Autodesk Inventor part; units mm, degrees
ref_plane "YZ Plane" through (0, 0, 0) normal (1, 0, 0) x (0, 1, 0)
ref_plane "XZ Plane" through (0, 0, 0) normal (0, 1, 0) x (-1, 0, 0)
ref_plane "XY Plane" through (0, 0, 0) normal (0, 0, 1) x (1, 0, 0)
sketch "Sketch1" plane through (0, 0, 0) normal (1, 0, 0) x (0, 1, 0)
  line L0 (0, 0) -> (22.86, 0)
  line L1 (22.86, 0) -> (22.86, -22.86)
  line L2 (22.86, -22.86) -> (0, -22.86)
  line L3 (0, -22.86) -> (0, 0)
  line L4 (0, -22.86) -> (15.24, -22.86)
  line L5 (0, -22.86) -> (15.24, -22.86) construction
  line L6 (15.24, -22.86) -> (15.24, -27.94)
  line L7 (15.24, -27.94) -> (17.78, -27.94)
  line L8 (17.78, -27.94) -> (17.78, -22.86)
  line L9 (17.78, 0) -> (17.78, 5.08)
  line L10 (17.78, 5.08) -> (15.24, 5.08)
  line L11 (15.24, 5.08) -> (15.24, 0)
  line L12 (17.9128, 0) -> (15.0818, 0)
  line L13 (15.0818, 5.3336) -> (17.9128, 5.3336)
  line L14 (17.9128, -22.86) -> (15.0818, -22.86)
  line L15 (15.0818, -28.1853) -> (17.9128, -28.1853)
  line L16 (17.9128, 0.0837) -> (17.9128, 5.3336)
  line L17 (15.0818, 0.0837) -> (15.0818, 5.3336)
  line L18 (15.0818, 0.0837) -> (-0.2071, 0.0837)
  line L19 (-0.2071, 0.0837) -> (-0.2071, -23.0588)
  line L20 (-0.2071, -23.0588) -> (15.0818, -23.0588)
  line L21 (15.0818, -23.0588) -> (15.0818, -28.1853)
  line L22 (17.9128, -28.1853) -> (17.9128, -23.0588)
  line L23 (17.9128, -23.0588) -> (22.86, -23.0588)
  line L24 (22.86, -23.0588) -> (22.86, -29.4177)
  line L25 (22.86, -29.4177) -> (-6.35, -29.4177)
  line L26 (22.86, 0.0837) -> (17.9128, 0.0837)
  line L27 (22.86, 0.0837) -> (22.86, 6.4337)
  line L28 (22.86, 6.4337) -> (-6.35, 6.4337)
  line L29 (-6.35, -29.4177) -> (-6.35, 6.4337)
  dimension "d0" = 22.86
  dimension "d1" = 22.86
  dimension "d4" = 5.08
  dimension "d5" = 2.54
  dimension "d6" = 5.08
  dimension "d7" = 2.54
  dimension "d9" = 29.21
  dimension "d11" = 6.35
extrude "Extrusion1" add sketch "Sketch1" along normal blind 12.7 contours L17 L18 L19 L20 L21 L15 L22 L23 L24 L25 L29 L28 L27 L26 L16 L13
sketch "Sketch2" plane through (12.7, 0, 0) normal (1, 0, 0) x (0, 0, -1)
  line L0 (-6.4337, 22.86) -> (-6.4337, -6.35)
  line L1 (29.4177, 22.86) -> (23.0588, 22.86)
  line L2 (-6.4337, -6.35) -> (29.4177, -6.35)
  line L3 (29.4177, -6.35) -> (29.4177, 22.86)
  line L4 (29.4177, 22.86) -> (-6.4337, 22.86)
  line L5 (-6.4337, 22.86) -> (-6.4337, -6.35)
  point P0 (0, 0)
  dimension "d16" = 29.21
  dimension "d17" = 35.8513
extrude "Extrusion2" add sketch "Sketch2" along normal blind 2.54
sketch "Sketch3" plane through (0, 0, 0) normal (-1, 0, 0) x (0, 0, 1)
  line L0 (-29.4177, -6.35) -> (-29.4177, 22.86)
  line L1 (6.4337, -6.35) -> (-29.4177, -6.35)
  line L2 (-29.4177, 0) -> (6.4337, 0)
  line L3 (6.4337, 0) -> (6.4337, -6.35)
  line L4 (6.4337, -6.35) -> (-29.4177, -6.35)
  line L5 (-29.4177, -6.35) -> (-29.4177, 0)
  point P0 (0, 0)
extrude "Extrusion3" add sketch "Sketch3" along normal blind 25.4
sketch "Sketch4" plane through (-25.4, 0, 0) normal (-1, 0, 0) x (0, 0, 1)
  line L0 (6.4337, -6.35) -> (-29.4177, -6.35)
  line L1 (6.4337, 22.86) -> (6.4337, -6.35)
  line L2 (-29.4177, -6.35) -> (6.4337, -6.35)
  line L3 (6.4337, -6.35) -> (6.4337, 22.86)
  line L4 (-29.4177, 22.86) -> (-29.4177, -6.35)
  line L5 (6.4337, 32.258) -> (-29.4177, 32.258)
  line L6 (-29.4177, 32.258) -> (-29.4177, 22.86)
  line L7 (-29.4177, 32.258) -> (-7.1927, 32.258)
  line L8 (-7.1927, 32.258) -> (-11.6377, 32.258)
  line L9 (-29.4177, 22.86) -> (6.4337, 22.86)
  line L10 (-11.6377, 32.258) -> (-9.4152, 32.258)
  line L11 (-9.4152, 22.86) -> (-11.6377, 22.86)
  line L12 (-9.4152, 22.86) -> (-13.8602, 22.86)
  line L13 (-13.8602, 22.86) -> (-13.8602, 32.258)
  line L14 (-13.8602, 32.258) -> (-9.4152, 32.258)
  line L15 (-27.8895, 28.6463) -> (-14.6164, 28.6463)
  line L16 (-14.6164, 28.6463) -> (-14.6164, 25.8191)
  line L17 (-14.6164, 25.8191) -> (-27.8895, 25.8191)
  line L18 (-27.8895, 25.8191) -> (-27.8895, 28.6463)
  line L19 (-8.2851, 28.6463) -> (5.4248, 28.6463)
  line L20 (5.4248, 28.6463) -> (5.4248, 25.8191)
  line L21 (5.4248, 25.8191) -> (-8.2851, 25.8191)
  line L22 (-8.2851, 25.8191) -> (-8.2851, 28.6463)
  line L23 (-8.2851, 28.6463) -> (5.4248, 28.6463)
  line L24 (5.4248, 28.6463) -> (5.4248, 25.8191)
  line L25 (5.4248, 25.8191) -> (-8.2851, 25.8191)
  line L26 (-8.2851, 25.8191) -> (-8.2851, 28.6463)
  line L27 (6.4337, 32.258) -> (-9.4152, 32.258)
  line L28 (-9.4152, 32.258) -> (-9.4152, 22.86)
  line L29 (-9.4152, 22.86) -> (6.4337, 22.86)
  line L30 (6.4337, 22.86) -> (6.4337, 32.258)
  line L31 (-29.4177, -6.35) -> (-29.4177, 22.86)
  line L32 (0.0837, 22.86) -> (6.4337, 22.86)
  line L33 (-29.4177, 22.86) -> (6.4337, 22.86)
  line L34 (6.4337, 22.86) -> (6.4337, 32.258)
  line L35 (6.4337, 32.258) -> (-29.4177, 32.258)
  line L36 (-29.4177, 22.86) -> (-29.4177, 32.258)
  point P0 (0, 0)
  dimension "d21" = 22.225
  dimension "d23" = 2.2225
  dimension "d24" = 4.445
extrude "Extrusion7" add sketch "Sketch4" along normal blind 12.7 contours L0 L4 L9 L1 | L9 L28 L5 L30 | L6 L5 L13 L9
sketch "Sketch6" plane through (-25.4, 32.258, -13.8602) normal (0, 1, 0) x (1, 0, 0)
  line L0 (0, 15.5575) -> (-12.7, 15.5575)
  line L1 (0, -20.2938) -> (-12.7, -20.2938)
  line L2 (-12.7, 15.5575) -> (0, 15.5575)
  line L3 (0, 15.5575) -> (0, -20.2938)
  line L4 (0, -20.2938) -> (-12.7, -20.2938)
  line L5 (-12.7, -20.2938) -> (-12.7, 15.5575)
  point P0 (25.4, -13.8602)
extrude "Extrusion8" add sketch "Sketch6" along normal blind 2.54
sketch "Sketch7" plane through (0, 22.86, 6.4337) normal (0, 0, 1) x (1, 0, 0)
  line L0 (0, 0) -> (15.24, 0)
  line L1 (-38.1, -29.21) -> (-38.1, 11.938)
  line L2 (15.24, 0) -> (-38.1, 0)
  line L3 (-38.1, 0) -> (-38.1, -29.21)
  line L4 (-38.1, -29.21) -> (15.24, -29.21)
  line L5 (15.24, -29.21) -> (15.24, 0)
  point P0 (0, -22.86)
extrude "Extrusion9" add sketch "Sketch7" along normal blind 2.54
sketch "Sketch8" plane through (0, 22.86, -23.0588) normal (0, 1, 0) x (1, 0, 0)
  line L0 (15.24, -32.0324) -> (-38.1, -32.0324)
  line L1 (-12.8761, -32.0324) -> (9.9839, -32.0324)
  line L2 (-12.8761, -47.2724) -> (-12.8761, -32.0324)
  line L3 (9.9839, -47.2724) -> (15.24, -47.2724)
  line L4 (15.24, -32.0324) -> (9.9839, -32.0324)
  line L5 (9.9839, -32.0324) -> (9.9839, -47.2724)
  line L6 (-12.8761, -47.2724) -> (-18.1339, -47.2724)
  line L7 (-18.1339, -32.0324) -> (-12.8761, -32.0324)
  line L8 (-12.8761, -32.0324) -> (-12.8761, -47.2724)
  line L9 (9.9839, -32.0324) -> (15.24, -32.0324)
  line L10 (15.24, -47.2724) -> (9.9839, -47.2724)
  line L11 (9.9839, -47.2724) -> (9.9839, -32.0324)
  line L12 (-18.1339, -32.0324) -> (15.24, -32.0324)
  line L13 (15.24, -32.0324) -> (15.24, -47.2724)
  line L14 (15.24, -32.0324) -> (9.9839, -32.0324)
  line L15 (-18.1339, -47.2724) -> (-18.1339, -32.0324)
  line L16 (-12.8761, -32.0324) -> (-18.1339, -32.0324)
  point P0 (0, -23.0588)
  dimension "d37" = 22.86
  dimension "d39" = 5.2578
extrude "Extrusion11" add sketch "Sketch8" against normal blind 29.21
sketch "Sketch9" plane through (-18.1339, 22.86, 24.2137) normal (0, 0, 1) x (1, 0, 0)
  line L0 (5.2578, -29.21) -> (0, -29.21)
  line L1 (5.2578, 0) -> (5.2578, -29.21)
  line L2 (5.2578, -16.51) -> (28.0868, -16.51)
  line L3 (28.0868, -16.51) -> (28.0868, 0)
  line L4 (28.0868, 0) -> (5.2578, 0)
  line L5 (5.2578, 0) -> (5.2578, -16.51)
  point P0 (18.1339, -22.86)
  dimension "d44" = 12.7
extrude "Extrusion12" add sketch "Sketch9" against normal blind 15.5575
sketch "Sketch10" plane through (9.9839, 22.86, 8.9737) normal (-1, 0, 0) x (0, 0, 1)
  line L0 (1.8867, -18.3591) -> (13.634, -18.3591)
  line L1 (13.634, -18.3591) -> (13.634, -27.4569)
  line L2 (13.634, -27.4569) -> (1.8867, -27.4569)
  line L3 (1.8867, -27.4569) -> (1.8867, -18.3591)
  point P0 (-8.9737, -22.86)
extrude "Extrusion13" cut sketch "Sketch10" against normal blind 15.5575
sketch "Sketch11" plane through (15.24, 22.86, -29.4177) normal (0, 0, -1) x (-1, 0, 0)
  line L0 (3.4492, -12.7029) -> (13.9615, -12.7029)
  line L1 (13.9615, -12.7029) -> (13.9615, -21.6525)
  line L2 (13.9615, -21.6525) -> (3.4492, -21.6525)
  line L3 (3.4492, -21.6525) -> (3.4492, -12.7029)
  point P0 (15.24, -22.86)
extrude "Extrusion14" cut sketch "Sketch11" against normal blind 15.5575
properties part number "thingy_for_arms_servo"
The listing builds one solid part. Answer for the finished solid, in the listing's coordinates (mm). A direction names the side the tool comes from. Coordinates: 2 decimals unless noted, no trailing zeros. Write each loop counter-clockwise with the first axis right and the second up, starting at its lowest first coordinate (ties: lowest second). Pieces come first, ordered by that corner, then holes. Notation, with made-up numbers: (-26.5, 12.5) - (22.5, 12.5) arc R26 cw to (22.5, 34.5) - close; hole circle Ø11 at (79, 61). An arc over 180 degrees is marked (long way). Return JSON: item names as keys, results as strings. Group by question number.
Q1. The part is cut by section C-C on z = 14.5. Write down the section's boundary in (x, y), and give its area (3 significant figures).
Q2. For a pull along X with two mould halves and no side action, classify faces 1 (the flat face through (11.791, 6, -26)), 2 (the flat face through (15.24, 8, -3)), 3 (the flat face through (-12, -6.35, -9)) as +X half, -X half, draft (parallel to the pull), parting line (faces both ways), or undercut.
Q3. The part is cut by section D-D on z = -17. Write down the section's boundary in (x, y), and give its area (3 significant figures).
Q4. The part is cut by section B-B on y = -1. Write down the section's boundary in (x, z), and give its area (3 significant figures).
Q5. Which of the six approach directions +Z, -Z, +X, -X, +Y, -Y give full straight-line access (tool end or side, diameter ignored) to faces 4 (the flat face through (-32, 34, 6.434)), 5 (the flat face through (-13, 12, 6.434)), 6 (the flat face through (6, 17.913, 3))?
Q6. Find the intervals of material crossed by line 1 along X through (y, z) = (5, -24); line 2 along X through (y, z) = (15.5, 5.5); line 3 along Y through (x, z) = (5, -25.5), in increasing order. Write a range as [from, to].
Q7. The part is cut by section A-A on x = 5.5. Write down the section's boundary in (y, z), and give its area (3 significant figures).
Q8. Flat-ended cylindrical pins translate along their axes: pin 1 Ø4 at (x, z) = (6.5, 1.5) entering from +Y; pin 2 Ø2 at (x, y) = (-23.5, 17.5) entering from -Z; pin 3 Ø2 at (x, y) = (-25.5, 20) entering from +Z. Find the tip coordinate at first contact, or state that the pin passes through.
Evaluation:
{
 "1": {"outline": "(-18.13, -6.35) - (-12.88, -6.35) - (-12.88, 6.35) - (9.95, 6.35) - (9.95, 22.86) - (-18.13, 22.86) - close; (9.98, -6.35) - (15.24, -6.35) - (15.24, -4.6) - (9.98, -4.6) - close; (9.98, 4.5) - (15.24, 4.5) - (15.24, 22.86) - (9.98, 22.86) - close", "area": "636 mm2"},
 "2": {"face 1": "undercut", "face 2": "+X half", "face 3": "draft"},
 "3": {"outline": "(-38.1, -6.35) - (15.24, -6.35) - (15.24, 22.86) - (12.7, 22.86) - (12.7, -0.21) - (0, -0.21) - (0, 0) - (-25.4, 0) - (-25.4, 25.82) - (-38.1, 25.82) - close; (-38.1, 28.65) - (-25.4, 28.65) - (-25.4, 34.8) - (-38.1, 34.8) - close", "area": "800 mm2"},
 "4": {"outline": "(-38.1, -29.42) - (15.24, -29.42) - (15.24, 10.86) - (9.98, 10.86) - (9.98, 8.97) - (-12.88, 8.97) - (-12.88, 24.21) - (-18.13, 24.21) - (-18.13, 8.97) - (-38.1, 8.97) - close; (9.98, 22.61) - (15.24, 22.61) - (15.24, 24.21) - (9.98, 24.21) - close", "area": "2,150 mm2"},
 "5": {"face 4": "+Z, +X, -X, +Y", "face 5": "-Z, +Y", "face 6": "none"},
 "6": {"line 1": "x = [-38.1, -25.4], [0, 1.28], [11.79, 15.24]", "line 2": "x = [-38.1, -25.4], [0, 15.24]", "line 3": "y = [-6.35, 1.21], [10.16, 15.08], [17.91, 22.86]"},
 "7": {"outline": "(-6.35, -29.42) - (1.21, -29.42) - (1.21, -23.06) - (-0.21, -23.06) - (-0.21, 0.08) - (15.08, 0.08) - (15.08, 5.33) - (17.91, 5.33) - (17.91, 0.08) - (22.86, 0.08) - (22.86, 24.21) - (6.35, 24.21) - (6.35, 8.97) - (-6.35, 8.97) - close; (10.16, -29.42) - (22.86, -29.42) - (22.86, -23.06) - (17.91, -23.06) - (17.91, -28.19) - (15.08, -28.19) - (15.08, -23.06) - (10.16, -23.06) - close", "area": "753 mm2"},
 "8": {"pin 1": "stops at y = 22.86", "pin 2": "stops at z = 6.43", "pin 3": "stops at z = 8.97"}
}
